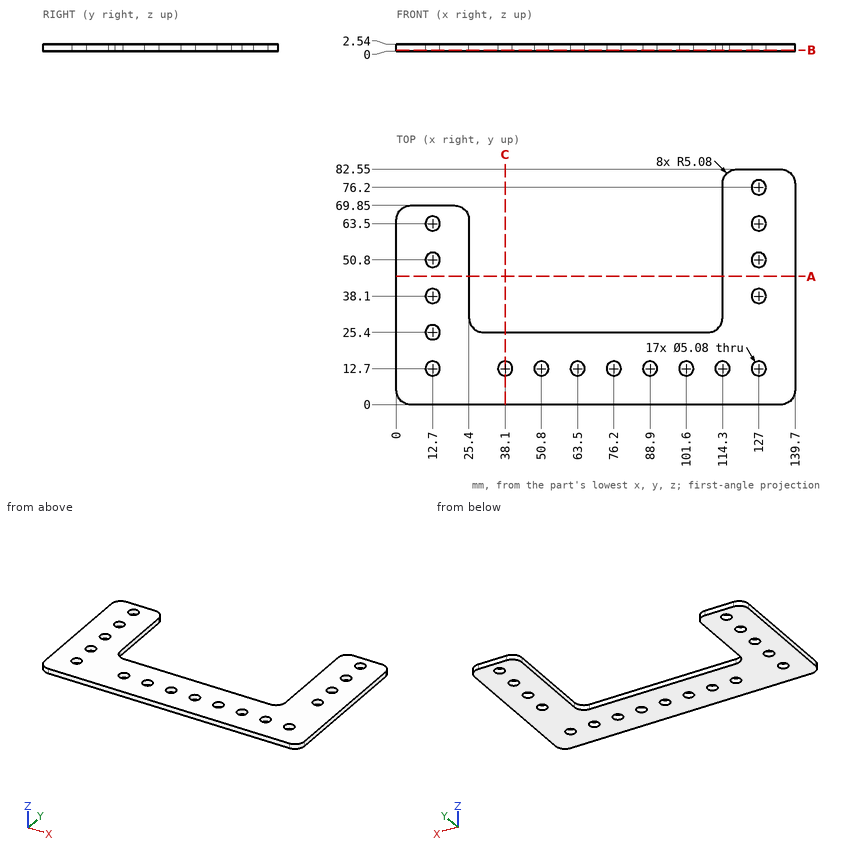
Design review of the part shown in the three views and the two pictorial views. Dimensions are in mm from the part's minimum x, y and z. Give positions to 0.01 mm unless a question says otherwise; leave off trailing zeros. Loops run counter-clockwise (first coordinate to the right, second up) from the corner with the lowest first, then second, coordinate; pieces in that order, holes last. Notation, with made-up numbers: M 46,2 L 84,2 A26 ccw 84,36 Z; hole C 80,33.5 d6. An arc over 180 degrees is marked long. Answer as a JSON object with one key per item and string values.
Item 1: We need section B-B (z = 0.4). Count the separate pieces of the cut face and the enclosed holes in it, and give its area (3 significant figures).
Output values:
{"separate pieces": "1", "enclosed holes": "17", "area": "5,760 mm2"}
Item 2: We need section C-C (x = 38.1). State the section outline as (y, z) points.
Output values:
{"outline": "M 0,0 L 10.16,0 L 10.16,2.54 L 0,2.54 Z; M 15.24,0 L 25.4,0 L 25.4,2.54 L 15.24,2.54 Z"}
Item 3: Wall thickness on line 1 along Y through (x, z) = (127, 1.8); line 2 along X through (y, z) = (50.5, 1.15); line 3 along Y through (x, z) = (12, 1.6): over which ranges is each line inside the solid? List them lowest first.
Output values:
{"line 1": "y = 0 to 10.16, 15.24 to 35.56, 40.64 to 48.26, 53.34 to 60.96, 66.04 to 73.66, 78.74 to 82.55", "line 2": "x = 0 to 10.18, 15.22 to 25.4, 114.3 to 124.48, 129.52 to 139.7", "line 3": "y = 0 to 10.26, 15.14 to 22.96, 27.84 to 35.66, 40.54 to 48.36, 53.24 to 61.06, 65.94 to 69.85"}
Item 4: We need section A-A (y = 45). State the section outline as (x, z) points.
Output values:
{"outline": "M 0,0 L 25.4,0 L 25.4,2.54 L 0,2.54 Z; M 114.3,0 L 139.7,0 L 139.7,2.54 L 114.3,2.54 Z"}
Item 5: For P1, Ø0.8, axis at y = 65.5, z = 1, coming from the -X side; P2, Ø3, axis at x = 127, y = 38.1, coming from the -Z side, all flat-tipped, find the tip position at first contact; note any pin that passes through.
Output values:
{"P1": "stops at x = 0.01", "P2": "passes through"}
